```python
from build123d import *

# Parameters (mm, degrees)
SKETCH2_W                       = 20
SKETCH2_H                       = 10
BOSS_EXTRUDE1_DEPTH             = 5.8
CHAMFER1_SIZE                   = 9.5
CHAMFER1_SIZE2                  = 8.553838421
FILLET3_R                       = 1
SKETCH3_W                       = 20
SKETCH3_H                       = 20
BOSS_EXTRUDE2_DEPTH             = 3
BOSS_EXTRUDE3_REACH             = 22.061
SKETCH6_R                       = 10
SKETCH6_R_2                     = 7
BOSS_EXTRUDE3_DIRECTION_2_REACH = 22.061
BOSS_EXTRUDE4_REACH             = 31.381
BOSS_EXTRUDE4_END_RADIUS        = 10
SKETCH5_W                       = 5
SKETCH5_H                       = 16
CUT_EXTRUDE1_REACH              = 35.977
CUT_EXTRUDE1_END_RADIUS         = 10
SKETCH7_R                       = 2.25


with BuildPart() as part:
    # Sketch2 → Boss-Extrude1 (new, symmetric)
    with BuildSketch(Plane.XY):
        Rectangle(SKETCH2_W, SKETCH2_H)
    extrude(amount=BOSS_EXTRUDE1_DEPTH, both=True)

    # Chamfer1
    chamfer1_edges = [part.edges().sort_by_distance(p)[0] for p in [
        (-10, 5, 0),
        (10, 5, 0),
    ]]
    chamfer1_side = [part.faces().sort_by_distance(p)[0] for p in [
        (0, 5, 0),
    ]]
    chamfer(chamfer1_edges, length=CHAMFER1_SIZE, length2=CHAMFER1_SIZE2, reference=chamfer1_side[0])

    # Fillet3
    fillet3_edges = [part.edges().sort_by_distance(p)[0] for p in [
        (-0.5, 5, 0),
        (0.5, 5, 0),
        (10, -3.553838421, 0),
        (-10, -3.553838421, 0),
    ]]
    fillet(fillet3_edges, radius=FILLET3_R)

    # Sketch3 → Boss-Extrude2 (add)
    with BuildSketch(Plane.XY.offset(5.8)):
        with Locations((0, 5)):
            Rectangle(SKETCH3_W, SKETCH3_H)
    boss_extrude2 = extrude(amount=BOSS_EXTRUDE2_DEPTH)

    # Mirror1: Boss-Extrude2 across plane
    add(boss_extrude2.mirror(Plane.XY))


with BuildPart() as body_2:

    # Boss-Extrude3: up to this face of the body (flat: up to its plane)
    boss_extrude3_end = Plane(part.part.faces().sort_by_distance((0, 15, 7.3))[0])
    # Sketch6 → Boss-Extrude3 (new, up to the picked face)
    with BuildSketch(Plane(origin=(0, 0, 0), x_dir=(1, 0, 0), z_dir=(0, 1, 0)), mode=Mode.PRIVATE) as boss_extrude3_sk1:
        with Locations(Location((0, -22, 0), (0, 0, 90))):
            Circle(SKETCH6_R)
        with Locations(Location((0, -22, 0), (0, 0, 90))):
            Circle(SKETCH6_R_2, mode=Mode.SUBTRACT)
    boss_extrude3_tool1 = split(extrude(boss_extrude3_sk1.sketch, amount=BOSS_EXTRUDE3_REACH, mode=Mode.PRIVATE), bisect_by=boss_extrude3_end, keep=Keep.BOTH, mode=Mode.PRIVATE)
    add(boss_extrude3_tool1.solids().sort_by(Axis((0, 0, 31.717157), (0, 1, 0)))[0])


    # Boss-Extrude3 direction 2: up to this face of the body (flat: up to its plane)
    boss_extrude3_direction_2_end = Plane(part.part.faces().sort_by_distance((0, -5, 0))[0])
    # Sketch6 → Boss-Extrude3 direction 2 (add, up to the picked face)
    with BuildSketch(Plane(origin=(0, 0, 0), x_dir=(1, 0, 0), z_dir=(0, 1, 0)), mode=Mode.PRIVATE) as boss_extrude3_direction_2_sk1:
        with Locations(Location((0, -22, 0), (0, 0, 90))):
            Circle(SKETCH6_R)
        with Locations(Location((0, -22, 0), (0, 0, 90))):
            Circle(SKETCH6_R_2, mode=Mode.SUBTRACT)
    boss_extrude3_direction_2_tool1 = split(extrude(boss_extrude3_direction_2_sk1.sketch, amount=-BOSS_EXTRUDE3_DIRECTION_2_REACH, mode=Mode.PRIVATE), bisect_by=boss_extrude3_direction_2_end, keep=Keep.BOTH, mode=Mode.PRIVATE)
    add(boss_extrude3_direction_2_tool1.solids().sort_by(Axis((0, 0, 31.717157), (0, -1, 0)))[0])


with BuildPart() as part_1:
    add(part.part)

    add(body_2.part)  # Boss-Extrude4 merges body 2
    # Boss-Extrude4: up to this cylinder (the profile starts outside it)
    boss_extrude4_end = Plane(origin=(0, 5, 22), z_dir=(0, -1, 0)) * Cylinder(BOSS_EXTRUDE4_END_RADIUS, 83.762, mode=Mode.PRIVATE)
    # Sketch5 → Boss-Extrude4 (add, up to the surface)
    with BuildSketch(Plane.XY.offset(8.8), mode=Mode.PRIVATE) as boss_extrude4_sk1:
        with Locations((0, 5)):
            Rectangle(SKETCH5_W, SKETCH5_H)
    boss_extrude4_tool1 = extrude(boss_extrude4_sk1.sketch, amount=BOSS_EXTRUDE4_REACH, mode=Mode.PRIVATE) - boss_extrude4_end
    add(boss_extrude4_tool1.solids().sort_by_distance((0, 5, 8.8))[0])

    # Cut-Extrude1: up to this cylinder (the profile starts inside it)
    cut_extrude1_end = Plane(origin=(0, 5, 22), z_dir=(0, -1, 0)) * Cylinder(CUT_EXTRUDE1_END_RADIUS, 103.954, mode=Mode.PRIVATE)
    # Sketch7 → Cut-Extrude1 (cut, up to the surface)
    with BuildSketch(Plane.XY.offset(20), mode=Mode.PRIVATE) as cut_extrude1_sk1:
        with Locations(Location((0, 10.5, 0), (0, 0, 180))):
            Circle(SKETCH7_R)
    cut_extrude1_tool1 = extrude(cut_extrude1_sk1.sketch, amount=CUT_EXTRUDE1_REACH, mode=Mode.PRIVATE) & cut_extrude1_end
    add(cut_extrude1_tool1.solids().sort_by_distance((0, 10.5, 20))[0], mode=Mode.SUBTRACT)
    # Sketch7 → Cut-Extrude1 (cut, up to the surface)
    with BuildSketch(Plane.XY.offset(20), mode=Mode.PRIVATE) as cut_extrude1_sk2:
        with Locations(Location((0, -0.5, 0), (0, 0, 180))):
            Circle(SKETCH7_R)
    cut_extrude1_tool2 = extrude(cut_extrude1_sk2.sketch, amount=CUT_EXTRUDE1_REACH, mode=Mode.PRIVATE) & cut_extrude1_end
    add(cut_extrude1_tool2.solids().sort_by_distance((0, -0.5, 20))[0], mode=Mode.SUBTRACT)


solid = part_1.part
```
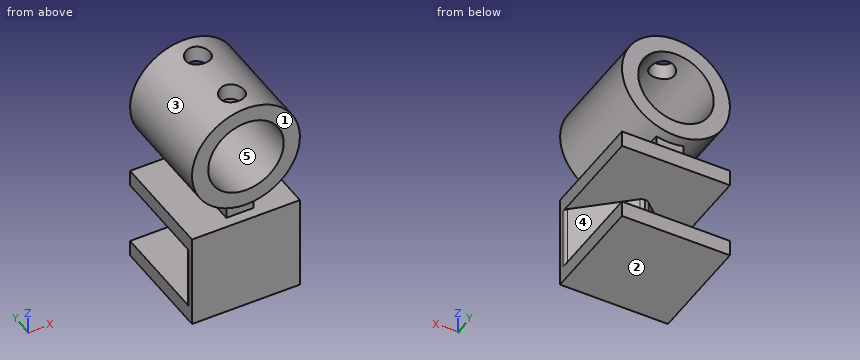
The listing builds one solid part. Answer for the finished solid, in the listing's coordinates (mm). Face numbers are marked on the shaded views. A direction names the side the tool comes from. Coordinates: 2 decimals unless noted, no trailing zeros. Loops run counter-clockwise (first coordinate to the right, second up) from the corner with the lowest first, then second, coordinate; pieces in that order, holes last. Notation, with made-up numbers: (14, 33.25) -> (35, 33.25) arc R31 cw to (35, 64.25) -> close; hole circle Ø11 at (18, 41.25). An arc over 180 degrees is marked (long way). Return JSON: item names as keys, results as strings. Group by question number.
(1) A cutting plane is placed at B-B on y = 11. Write down the section's boundary in (x, z).
(2) Determine the mould class of the marked faces 1, 2 and 3 for opening direction Z: released by +Z, released by -Z, zero draft, split by the parting line, or undercut.
(3) Given pin 1 Ø4 at (x, z) = (1, 17.5) entering from -Y; pin 2 Ø2 at (y, z) = (9, 15.5) entering from +X; pin 3 Ø8 at (x, y) = (6, 10.5) entering from +Z; pin 4 Ø8 at (y, z) = (2, 13.5) entering from +X, each flat-ended and moving along its own axis, determine where each tip first touches the part or whether it passes through.
(4) A cutting plane is placed at D-D on y = -0.5. Write down the section's boundary in (x, z).
(5) A cutting plane is placed at C-C on x = -6. Write down the section's boundary in (y, z), and give its area (3 significant figures).
(6) Which of the six approach directions +Z, -Z, +X, -X, +Y, -Y give full straight-line access (tool end or side, diameter ignored) to the marked faces 4 and 5?
(7) A cutting plane is placed at A-A on z = 22. Write down the section's boundary in (x, y).
(8) Find the intervals of material crossed by probe 1 along Y at (x, z) = (-2, 29); probe 2 along Z at (x, y) = (-4.25, 5.75); probe 3 along X at (y, z) = (8.75, 22), in increasing order. Write a range as from..to.
The answers:
{
 "1": {"outline": "(-10, -8.8) -> (10, -8.8) -> (10, -5.8) -> (-10, -5.8) -> close; (-10, 5.8) -> (10, 5.8) -> (10, 8.8) -> (2.5, 8.8) -> (2.5, 12.32) arc R10 ccw to (2.19, 31.76) -> (2.19, 28.65) arc R7 cw (long way) to (-2.19, 28.65) -> (-2.19, 31.76) arc R10 ccw to (-2.5, 12.32) -> (-2.5, 8.8) -> (-10, 8.8) -> close"},
 "2": {"face 1": "zero draft", "face 2": "released by -Z", "face 3": "undercut"},
 "3": {"pin 1": "passes through", "pin 2": "stops at x = 8.35", "pin 3": "stops at z = 31.78", "pin 4": "stops at x = 8.93"},
 "4": {"outline": "(-10, -8.8) -> (10, -8.8) -> (10, -5.8) -> (6.61, -5.8) -> (6.61, 5.8) -> (10, 5.8) -> (10, 8.8) -> (2.5, 8.8) -> (2.5, 12.32) arc R10 ccw to (2.25, 31.74) -> (2.25, 28.63) arc R7 cw (long way) to (-2.25, 28.63) -> (-2.25, 31.74) arc R10 ccw to (-2.5, 12.32) -> (-2.5, 8.8) -> (-10, 8.8) -> (-10, 5.8) -> (-6.61, 5.8) -> (-6.61, -5.8) -> (-10, -5.8) -> close"},
 "5": {"outline": "(-5, -8.8) -> (15, -8.8) -> (15, -5.8) -> (0.05, -5.8) -> (0.05, 5.8) -> (15, 5.8) -> (15, 8.8) -> (-5, 8.8) -> close; (-5, 14) -> (15, 14) -> (15, 18.39) -> (-5, 18.39) -> close; (-5, 25.61) -> (15, 25.61) -> (15, 30) -> (-5, 30) -> close", "area": "354 mm^2"},
 "6": {"face 4": "+X, +Y", "face 5": "+Y, -Y"},
 "7": {"outline": "(-10, -5) -> (-7, -5) -> (-7, 15) -> (-10, 15) -> close; (7, -5) -> (10, -5) -> (10, 15) -> (7, 15) -> close"},
 "8": {"probe 1": "y = -5..-1.53, 0.53..9.47, 11.53..15", "probe 2": "z = -8.8..-5.8, 5.8..8.8, 12.95..16.44, 27.56..31.05", "probe 3": "x = -10..-7, 7..10"}
}
